Design review of the part built by this model. Coordinates are the model's own, in mm. A direction names the side the tool comes from. Give positions to 0.01 mm unless a question says otherwise; leave off trailing zeros. Write each loop counter-clockwise with the first axis right and the second up, starting at its lowest first coordinate (ties: lowest second). Pieces come first, ordered by that corner, then holes. Notation, with made-up numbers: (62, 40.25) -> (70, 40.25) arc R13 cw to (70, 58.25) -> close; hole circle Ø7 at (29, -27). An arc over 180 degrees is marked (long way). Answer as a JSON object with one key per item and string values.
```python
from build123d import *

# Parameters (mm, degrees)
BOSS_EXTRUDE1_DEPTH = 10
SKETCH5_W           = 19.832190572
SKETCH5_H           = 38.694970839
BOSS_EXTRUDE2_DEPTH = 88.9
SKETCH6_R           = 22
SKETCH6_R_2         = 18.35
BOSS_EXTRUDE5_DEPTH = 5
FILLET8_R           = 2.5
FILLET10_R          = 2.5


# Some blends are built 0.0001 mm under size
with BuildPart() as part:
    # Sketch1 → Boss-Extrude1 (new body)
    with BuildSketch(Plane(origin=(0, 0, 0), x_dir=(1, 0, 0), z_dir=(0, 1, 0))):
        with BuildLine():
            Line((0, 22.182836405), (0, 38.694970839))
            Line((0, 38.694970839), (147.830868253, 38.694970839))
            Line((147.830868253, 38.694970839), (147.830868253, 0))
            Line((147.830868253, 0), (0, 0))
            Line((0, 0), (0, 16.512134434))
            add(Edge.make_bspline(
                [(0, 16.512134434), (3.388756459, 25.554510726), (4.766553868, 6.635260128), (7.812405429, 19.34748542)],
                knots=[0, 0, 0, 0, 1, 1, 1, 1], degree=3))
            add(Edge.make_bspline(
                [(0, 22.182836405), (3.388756459, 13.140460113), (4.562234719, 33.060495119), (7.812405429, 19.34748542)],
                knots=[0, 0, 0, 0, 1, 1, 1, 1], degree=3))
        make_face()
    extrude(amount=BOSS_EXTRUDE1_DEPTH)

    # Sketch5 → Boss-Extrude2 (add)
    with BuildSketch(Plane.XZ):
        with Locations((137.914772967, -19.347485419)):
            Rectangle(SKETCH5_W, SKETCH5_H)
    extrude(amount=BOSS_EXTRUDE2_DEPTH)

    # Sketch6 → Boss-Extrude5 (add)
    with BuildSketch(Plane.ZY.offset(-127.998677681)):
        with Locations(Location((-19.34748542, -65.278, 0), (0, 0, 151.573820003))):
            Circle(SKETCH6_R)
        with Locations((-19.34748542, -65.278)):
            Circle(SKETCH6_R_2, mode=Mode.SUBTRACT)
    extrude(amount=BOSS_EXTRUDE5_DEPTH)

    # Fillet8
    # the kernel refuses this fillet: 2.5 mm, written as the material it takes off along each edge
    with BuildSketch(Plane(origin=(122.998677681, -65.278, -19.34748542), x_dir=(0, 0.4760260947170219, -0.8794311554342733), z_dir=(0, 0.8794311554342733, 0.4760260947170219))) as fillet8_piece_1:
        with BuildLine():
            CenterArc((22 - FILLET8_R, -FILLET8_R), FILLET8_R, 0, 90)
            Line((22 - FILLET8_R, 0), (22, 0))
            Line((22, 0), (22, -FILLET8_R))
        make_face()
    revolve(axis=Axis((122.998677681, -65.278, -19.34748542), (-1, 0, 0)), mode=Mode.SUBTRACT)
    with BuildSketch(Plane(origin=(127.998677681, -65.278, -19.34748542), x_dir=(0, -0.7034691190214044, 0.7107258251838392), z_dir=(0, -0.7107258251838392, -0.7034691190214044))) as fillet8_piece_2_section:
        with BuildLine():
            CenterArc((22 - FILLET8_R, FILLET8_R), FILLET8_R, 270, 90)
            Line((22 - FILLET8_R, 0), (22, 0))
            Line((22, 0), (22, FILLET8_R))
        make_face()
    fillet8_piece_2 = revolve(axis=Axis((127.998677681, -65.278, -19.34748542), (-1, 0, 0)), revolution_arc=89.411997633, mode=Mode.PRIVATE)
    fillet8_piece_2 = split(fillet8_piece_2, bisect_by=Plane(origin=(127.287251046, -65.278, 0), z_dir=(0, 0, 1)), keep=Keep.TOP, mode=Mode.PRIVATE)
    add(fillet8_piece_2, mode=Mode.SUBTRACT)

    # Fillet10
    fillet10_edges = [part.edges().sort_by_distance(p)[0] for p in [
        (127.998677681, -65.278, -41.34748542),
    ]]
    fillet(fillet10_edges, radius=FILLET10_R - 0.0001)  # a hair under: the kernel refuses the full size


solid = part.part
```
(1) We need section A-A, the plane x = 43. State the section outline as (y, z) points.
Here are the results:
{"outline": "(0, -38.69) -> (10, -38.69) -> (10, 0) -> (0, 0) -> close"}
(2) For line 1 along Z through (x, y) = (89, 2); line 2 along Y through (x, z) = (88, -29); line 3 along X through (y, z) = (-31.5, -36), list the stretches that pass through material, from the lowest coordinate up.
Here are the results:
{"line 1": "z = -38.69 to 0", "line 2": "y = 0 to 10", "line 3": "x = 128 to 147.83"}
(3) For faces 1 (the flat face through (0, 5, -30)), 2 (the cylindrical face through (125.534, -59.766, -1.845)), 3 (the flat face through (122.999, -48, -27)), 4 (the flat face through (127.999, -88, -19)), list the 3-axis set-ups (+Z, -Z, +X, -X, +Y, -Y) from which the entire face can be reached by the end or side of a thin tool; tool diameter is ignored.
Here are the results:
{"face 1": "+Z, -Z, -X, +Y, -Y", "face 2": "-X", "face 3": "+Z, -Z, -X, -Y", "face 4": "-X, -Y"}
(4) Clearance check with flat-ended pins moving along their axes: pin 1 (11.5 mm diameter, centred on y = -59.5, z = -28, fed in from -X); pin 2 (19.5 mm diameter, centred on x = 92, z = -18, fed in from -Y); pin 3 (14.5 mm diameter, centred on y = -83, z = -12, fed in from -X). State where each tip first meets the part, or that it passes through.
Here are the results:
{"pin 1": "stops at x = 128", "pin 2": "stops at y = 0", "pin 3": "stops at x = 123"}
(5) We need section B-B, the plane y = -39. State the section outline as (x, z) points, then the cut area to 3 significant figures.
Here are the results:
{"outline": "(128, -38.69) -> (147.83, -38.69) -> (147.83, 0) -> (128, 0) -> close", "area": "767 mm²"}
